Read the model definition and answer for the solid it produces. Units are mm, in the model's axes. A direction names the side the tool comes from. Give positions to 0.01 mm unless a question says otherwise; leave off trailing zeros. Order: outer loops, then holes, each group sorted by start corner. A loop starts at its lowest first (then second) coordinate and runs counter-clockwise, first axis right, second up. Notation, with made-up numbers: (71, -11) -> (91, -11) arc R33 cw to (91, 28) -> close; hole circle Ø9 at (10.5, 19). An arc over 180 degrees is marked (long way). Answer as CSV lines item,"result". Start each with the question number.
1) Straight lines are drawn through the part: L1, parallel to X at y = 0.8, z = -9.5; L2, parallel to X at y = 6, z = -15; L3, parallel to Z at x = 93.5, y = 0.8. For each, find the intervals that lie inside material, in ascending order. Write a range as from..to.
2) Find section A-A (x = 2.6). Determine the outline of the cut face in (y, z), and give its area (3 significant figures).
3) Find section D-D (x = 39.5). Determine the outline of the cut face in (y, z), and give its area (3 significant figures).
4) Find section B-B (y = 6.5). Determine the outline of the cut face in (x, z), and give its area (3 significant figures).
5) Flat-ended cylindrical pins translate along their axes: pin 1 Ø5.5 at (x, y) = (52.5, 5) entering from -Z; pin 2 Ø4.5 at (x, z) = (12.5, -9.5) entering from +Y; pin 3 Ø2.5 at (x, y) = (82.5, 6.5) entering from -Z; pin 4 Ø5 at (x, z) = (28, -11) entering from -Y. Find the tip coordinate at first contact, or state that the pin passes through.
6) For faces 4 (the face through (47, 5, -19.6)), 5 (the face through (79.4, 5, -10)), 6 (the face through (47, 1, 0)), 7 (the face through (47, 5, -12.1)), 8 (the face through (12, 6, -15.4)), determine the directions among +Z, -Z, +X, -X, +Y, -Y from which every point of the face is accessible in a straight line to the end or side of a thin tool.
7) The mould has two halves that part along Z. Classify faces 1 (the face through (47, 1.5, -10)), 2 (the face through (77.3, 6, -16)), 3 (the face through (47, 5, -0.4)): +Z half, -Z half, draft (parallel to the pull), parting line (faces both ways), or undercut.
8) Find section C-C (z = -10). Determine the outline of the cut face in (x, y), and give its area (3 significant figures).
```python
from build123d import *
from OCP.BRepFilletAPI import BRepFilletAPI_MakeChamfer

# Parameters (mm, degrees)
SKETCH1_W                 = 96.1
SKETCH1_H                 = 20
SKETCH1_R                 = 1.5
BOSS_EXTRUDE1_DEPTH       = 1.5
SKETCH2_W                 = 60.1
SKETCH2_H                 = 7.5
BOSS_EXTRUDE2_DEPTH       = 10.1
CHAMFER1_SIZE             = 3
CHAMFER1_SIZE2            = 1.091910703
CHAMFER1_OF_MIRROR1_SIZE  = 3
CHAMFER1_OF_MIRROR1_SIZE2 = 1.091910703
SKETCH3_W                 = 7.6
SKETCH3_H                 = 10
BOSS_EXTRUDE3_DEPTH       = 9.8
CHAMFER2_SIZE             = 3
CHAMFER2_SIZE2            = 1.091910703


with BuildPart() as part:
    # Sketch1 → Boss-Extrude1 (new body)
    with BuildSketch(Plane(origin=(0, 0, 0), x_dir=(1, 0, 0), z_dir=(0, 1, 0))):
        with Locations((48.05, 10)):
            Rectangle(SKETCH1_W, SKETCH1_H)
        with Locations(Location((2.6, 9.5, 0), (0, 0, 270))):
            Circle(SKETCH1_R, mode=Mode.SUBTRACT)
        with Locations(Location((93.5, 9.5, 0), (0, 0, 270))):
            Circle(SKETCH1_R, mode=Mode.SUBTRACT)
    extrude(amount=BOSS_EXTRUDE1_DEPTH)

    # Sketch2 → Boss-Extrude2 (add)
    with BuildSketch(Plane(origin=(0, 1.5, 0), x_dir=(1, 0, 0), z_dir=(0, 1, 0))):
        with Locations((47.25, 4.15)):
            Rectangle(SKETCH2_W, SKETCH2_H)
    boss_extrude2 = extrude(amount=BOSS_EXTRUDE2_DEPTH)

    # Chamfer1: one chamfer whose edges measure the first distance from different faces: ONE call of the kernel's chamfer builder (chamfer() names one face for all edges)
    chamfer1_edges_1 = [part.edges().sort_by_distance(p)[0] for p in [
        (47.25, 11.6, -0.4),
    ]]
    chamfer1_side_1 = [part.faces().sort_by_distance(p)[0] for p in [
        (47.25, 6.55, -0.4),
    ]]
    chamfer1_edges_2 = [part.edges().sort_by_distance(p)[0] for p in [
        (47.25, 11.6, -7.9),
    ]]
    chamfer1_side_2 = [part.faces().sort_by_distance(p)[0] for p in [
        (47.25, 6.55, -7.9),
    ]]
    chamfer1 = BRepFilletAPI_MakeChamfer(part.part.solid().wrapped)
    for e in chamfer1_edges_1:
        chamfer1.Add(CHAMFER1_SIZE, CHAMFER1_SIZE2, e.wrapped, chamfer1_side_1[0].wrapped)  # the first distance lies on this face
    for e in chamfer1_edges_2:
        chamfer1.Add(CHAMFER1_SIZE, CHAMFER1_SIZE2, e.wrapped, chamfer1_side_2[0].wrapped)  # the first distance lies on this face
    add(Compound.cast(chamfer1.Shape()), mode=Mode.REPLACE)

    # Mirror1: Boss-Extrude2 across plane
    add(boss_extrude2.mirror(Plane.XY.offset(-10)))

    # Chamfer1 of Mirror1: one chamfer whose edges measure the first distance from different faces: ONE call of the kernel's chamfer builder (chamfer() names one face for all edges)
    chamfer1_of_mirror1_edges_1 = [part.edges().sort_by_distance(p)[0] for p in [
        (47.25, 11.6, -19.6),
    ]]
    chamfer1_of_mirror1_side_1 = [part.faces().sort_by_distance(p)[0] for p in [
        (47.25, 6.55, -19.6),
    ]]
    chamfer1_of_mirror1_edges_2 = [part.edges().sort_by_distance(p)[0] for p in [
        (47.25, 11.6, -12.1),
    ]]
    chamfer1_of_mirror1_side_2 = [part.faces().sort_by_distance(p)[0] for p in [
        (47.25, 6.55, -12.1),
    ]]
    chamfer1_of_mirror1 = BRepFilletAPI_MakeChamfer(part.part.solid().wrapped)
    for e in chamfer1_of_mirror1_edges_1:
        chamfer1_of_mirror1.Add(CHAMFER1_OF_MIRROR1_SIZE, CHAMFER1_OF_MIRROR1_SIZE2, e.wrapped, chamfer1_of_mirror1_side_1[0].wrapped)  # the first distance lies on this face
    for e in chamfer1_of_mirror1_edges_2:
        chamfer1_of_mirror1.Add(CHAMFER1_OF_MIRROR1_SIZE, CHAMFER1_OF_MIRROR1_SIZE2, e.wrapped, chamfer1_of_mirror1_side_2[0].wrapped)  # the first distance lies on this face
    add(Compound.cast(chamfer1_of_mirror1.Shape()), mode=Mode.REPLACE)

    # Sketch3 → Boss-Extrude3 (add)
    with BuildSketch(Plane(origin=(0, 1.5, 0), x_dir=(1, 0, 0), z_dir=(0, 1, 0))):
        with Locations((11.9, 10.4)):
            Rectangle(SKETCH3_W, SKETCH3_H)
        with Locations((83.2, 10.3)):
            Rectangle(SKETCH3_W, SKETCH3_H)
    extrude(amount=BOSS_EXTRUDE3_DEPTH)

    # Chamfer2: one chamfer whose edges measure the first distance from different faces: ONE call of the kernel's chamfer builder (chamfer() names one face for all edges)
    chamfer2_edges_1 = [part.edges().sort_by_distance(p)[0] for p in [
        (8.1, 11.3, -10.4),
    ]]
    chamfer2_side_1 = [part.faces().sort_by_distance(p)[0] for p in [
        (8.1, 6.4, -10.4),
    ]]
    chamfer2_edges_2 = [part.edges().sort_by_distance(p)[0] for p in [
        (15.7, 11.3, -10.4),
    ]]
    chamfer2_side_2 = [part.faces().sort_by_distance(p)[0] for p in [
        (15.7, 6.4, -10.4),
    ]]
    chamfer2_edges_3 = [part.edges().sort_by_distance(p)[0] for p in [
        (79.4, 11.3, -10.3),
    ]]
    chamfer2_side_3 = [part.faces().sort_by_distance(p)[0] for p in [
        (79.4, 6.4, -10.3),
    ]]
    chamfer2_edges_4 = [part.edges().sort_by_distance(p)[0] for p in [
        (87, 11.3, -10.3),
    ]]
    chamfer2_side_4 = [part.faces().sort_by_distance(p)[0] for p in [
        (87, 6.4, -10.3),
    ]]
    chamfer2 = BRepFilletAPI_MakeChamfer(part.part.solid().wrapped)
    for e in chamfer2_edges_1:
        chamfer2.Add(CHAMFER2_SIZE, CHAMFER2_SIZE2, e.wrapped, chamfer2_side_1[0].wrapped)  # the first distance lies on this face
    for e in chamfer2_edges_2:
        chamfer2.Add(CHAMFER2_SIZE, CHAMFER2_SIZE2, e.wrapped, chamfer2_side_2[0].wrapped)  # the first distance lies on this face
    for e in chamfer2_edges_3:
        chamfer2.Add(CHAMFER2_SIZE, CHAMFER2_SIZE2, e.wrapped, chamfer2_side_3[0].wrapped)  # the first distance lies on this face
    for e in chamfer2_edges_4:
        chamfer2.Add(CHAMFER2_SIZE, CHAMFER2_SIZE2, e.wrapped, chamfer2_side_4[0].wrapped)  # the first distance lies on this face
    add(Compound.cast(chamfer2.Shape()), mode=Mode.REPLACE)


solid = part.part
```
Findings below:
1,L1,"0..1.1, 4.1..92, 95..96.1"
1,L2,"8.1..15.7, 17.2..77.3, 79.4..87"
1,L3,"-20..-11, -8..0"
2,outline,"(0, -20) -> (1.5, -20) -> (1.5, -11) -> (0, -11) -> close; (0, -8) -> (1.5, -8) -> (1.5, 0) -> (0, 0) -> close"
2,area,"25.5 mm²"
3,outline,"(0, -20) -> (1.5, -20) -> (1.5, -19.6) -> (8.6, -19.6) -> (11.6, -18.51) -> (11.6, -13.19) -> (8.6, -12.1) -> (1.5, -12.1) -> (1.5, -7.9) -> (8.6, -7.9) -> (11.6, -6.81) -> (11.6, -1.49) -> (8.6, -0.4) -> (1.5, -0.4) -> (1.5, 0) -> (0, 0) -> close"
3,area,"175 mm²"
4,outline,"(8.1, -15.4) -> (15.7, -15.4) -> (15.7, -5.4) -> (8.1, -5.4) -> close; (17.2, -19.6) -> (77.3, -19.6) -> (77.3, -12.1) -> (17.2, -12.1) -> close; (17.2, -7.9) -> (77.3, -7.9) -> (77.3, -0.4) -> (17.2, -0.4) -> close; (79.4, -15.3) -> (87, -15.3) -> (87, -5.3) -> (79.4, -5.3) -> close"
4,area,"1,050 mm²"
5,pin 1,"z = -19.6"
5,pin 2,"y = 11.3"
5,pin 3,"z = -15.3"
5,pin 4,"y = 0"
6,face 4,"-Z, +X, -X, +Y"
6,face 5,"+Z, -Z, +Y"
6,face 6,"+Z, +X, -X, +Y, -Y"
6,face 7,"+Y"
6,face 8,"-Z, -X, +Y"
7,face 1,"undercut"
7,face 2,"draft"
7,face 3,"+Z half"
8,outline,"(0, 0) -> (1.19, 0) -> (1.19, 1.5) -> (0, 1.5) -> close; (4.01, 0) -> (92.09, 0) -> (92.09, 1.5) -> (87, 1.5) -> (87, 8.3) -> (85.91, 11.3) -> (80.49, 11.3) -> (79.4, 8.3) -> (79.4, 1.5) -> (15.7, 1.5) -> (15.7, 8.3) -> (14.61, 11.3) -> (9.19, 11.3) -> (8.1, 8.3) -> (8.1, 1.5) -> (4.01, 1.5) -> close; (94.91, 0) -> (96.1, 0) -> (96.1, 1.5) -> (94.91, 1.5) -> close"
8,area,"278 mm²"
